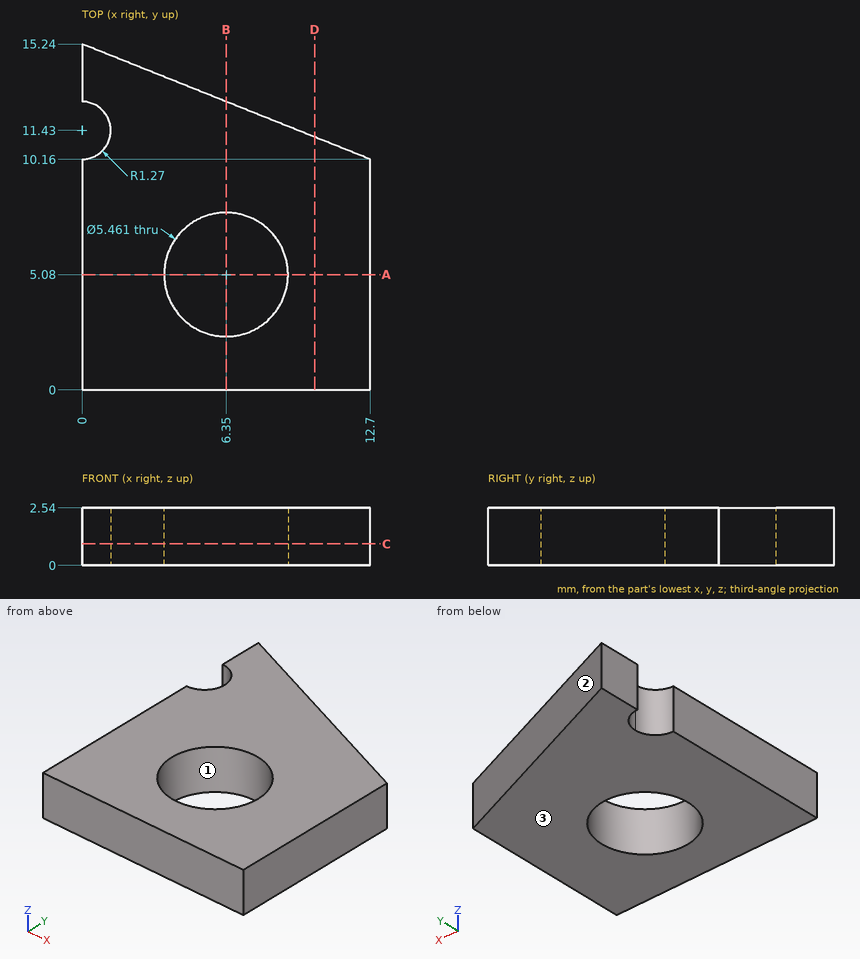
Input: dimensioned drawing with shaded views. Units: mm. Origin: part minimum x, y, z. Coordinates: 2 decimals unless noted, no trailing zeros. Order: outer loops, then holes, each group sorted by start corner. A loop starts at its lowest first (then second) coordinate and runs counter-clockwise, first axis right, second up. Notation, with made-up numbers: (-22.5, 83) - (-5.5, 83) arc R21 cw to (-5.5, 88) - close; hole circle Ø2 at (20.5, 15.5). An arc over 180 degrees is marked (long way). Return JSON: item names as keys, results as strings. Group by question number.
1. Cut plane A-A (y = 5.08). Output: boundary loops of the cut face in (x, z), plus the area to 3 significant figures.
2. Cut plane D-D (x = 10.25). Output: boundary loops of the cut face in (y, z), plus the area to 3 significant figures.
3. Material intervals for line 1 along Y through (x, z) = (6.35, 1.85); line 2 along Y through (x, z) = (4.75, 1.6); line 3 along X through (y, z) = (4.75, 0.4), sorted ascending. Write a range as [from, to].
4. Cut plane C-C (z = 0.95). Output: boundary loops of the cut face in (x, y).
5. Pull-direction query (Y, two-part tool) for the marked faces 1, 2 and 3; classes: pulls with the +Y half, pulls with the -Y half, needs draft (parallel to the pull), parting line crosses it, or undercut.
6. Cut plane B-B (x = 6.35). Output: boundary loops of the cut face in (y, z).
7. Pin query (flat end, axial travel): pin 1 (1.5 mm diameter, centred on x = 8, z = 1, fed in from +Y); pin 2 (6.5 mm diameter, centred on x = 6.35, y = 5.08, fed in from -Z). Return the tip coordinate at first contact, or that it passes through.
Resolved:
{
 "1": {"outline": "(0, 0) - (3.62, 0) - (3.62, 2.54) - (0, 2.54) - close; (9.08, 0) - (12.7, 0) - (12.7, 2.54) - (9.08, 2.54) - close", "area": "18.4 mm²"},
 "2": {"outline": "(0, 0) - (11.14, 0) - (11.14, 2.54) - (0, 2.54) - close", "area": "28.3 mm²"},
 "3": {"line 1": "y = [0, 2.35], [7.81, 12.7]", "line 2": "y = [0, 2.87], [7.29, 13.34]", "line 3": "x = [0, 3.64], [9.06, 12.7]"},
 "4": {"outline": "(0, 0) - (12.7, 0) - (12.7, 10.16) - (0, 15.24) - (0, 12.7) arc R1.27 cw to (1.27, 11.43) arc R1.27 cw to (0, 10.16) - close; hole circle Ø5.46 at (6.35, 5.08)"},
 "5": {"face 1": "undercut", "face 2": "pulls with the +Y half", "face 3": "needs draft"},
 "6": {"outline": "(0, 0) - (2.35, 0) - (2.35, 2.54) - (0, 2.54) - close; (7.81, 0) - (12.7, 0) - (12.7, 2.54) - (7.81, 2.54) - close"},
 "7": {"pin 1": "stops at y = 12.34", "pin 2": "stops at z = 0"}
}
